Read the model definition and answer for the solid it produces. Units are mm, in the model's axes. A direction names the side the tool comes from. Give positions to 0.01 mm unless a question says otherwise; leave off trailing zeros. Loops run counter-clockwise (first coordinate to the right, second up) from the corner with the lowest first, then second, coordinate; pieces in that order, holes last. Notation, with made-up numbers: (-36.75, -34) - (17.25, -34) arc R13 ccw to (17.25, -21) - close; hole circle Ø1 at (8, 31). An arc over 180 degrees is marked (long way). Put each result on its own line as item: value. Start each with the question number.
1. Consider L1, parallel to X at y = -2.5, z = 5.1; L2, parallel to X at y = -17, z = 2.75; L3, parallel to X at y = -13, z = 0.95. Determine where each line is inside the solid, lowest interval first. Write a range as from..to.
2. For a pull along Y with two mould halves and no side action, classify faces 1 (the cylindrical face through (-15.43, 15.63, 0.74)), 2 (the flat face through (-12, 12, 0)) as released by +Y, released by -Y, zero draft, split by the parting line, or undercut.
3. For faces 3 (the cylindrical face through (14.151, -11.046, 3.782)), 4 (the cylindrical face through (-1.852, -21.386, 3.042)), determine the directions among +Z, -Z, +X, -X, +Y, -Y from which every point of the face is accessible in a straight line to the end or side of a thin tool.
4. Given pin 1 Ø12 at (x, y) = (-14, 8) entering from -Z; pin 2 Ø3.5 at (x, y) = (13.28, -14.95) entering from +Z; pin 3 Ø3 at (y, z) = (16.5, 4.5) entering from -X; pin 4 Ø1.5 at (y, z) = (5, 3) entering from +X, each flat-ended and moving along its own axis, determine where each tip first touches the part or whether it passes through.
5. A cutting plane is placed at B-B, the plane z = 4.3. Count the separate pieces of the cut face and the enclosed holes in it, plus the area to 3 significant figures.
6. A cutting plane is placed at A-A, the plane x = -14. Determine the outline of the cut face in (y, z), plus the area to 3 significant figures.
```python
from build123d import *

# Parameters (mm, degrees)
ESQUISSE5_R                                     = 27
ESQUISSE5_R_2                                   = 15
BASE_EXTRUSION_DEPTH                            = 6
TROU_TARAUD_M4X0_71_D                           = 3.3
R_P_TITION_CIRCULAIRE1_COUNT                    = 4
CHAMBRAGE_POUR_VIS_T_TE_CYLINDRIQUE_D           = 4.5
CHAMBRAGE_POUR_VIS_T_TE_CYLINDRIQUE_CBORE_D     = 8
CHAMBRAGE_POUR_VIS_T_TE_CYLINDRIQUE_CBORE_DEPTH = 4.5
R_P_TITION_CIRCULAIRE2_COUNT                    = 6


with BuildPart() as part:
    # Esquisse5 → Base-Extrusion (new body)
    with BuildSketch(Plane.XY):
        with Locations(Location((0, 0, 0), (0, 0, 180))):
            Circle(ESQUISSE5_R)
        with Locations(Location((0, 0, 0), (0, 0, 180))):
            Circle(ESQUISSE5_R_2, mode=Mode.SUBTRACT)
    extrude(amount=BASE_EXTRUSION_DEPTH)

    # Trou taraudé M4x0.71 (through all)
    with Locations(Plane(origin=(0, 0, 0), x_dir=(-1, 0, 0), z_dir=(0, 0, -1))):
        with Locations((22.959989216, 1.356058707)):
            trou_taraud_m4x0_71 = Hole(TROU_TARAUD_M4X0_71_D / 2)

    # Répétition circulaire1: Trou taraudé M4x0.71 ×4 about axis
    r_p_tition_circulaire1_axis = Axis((0, 0, 0), (0, 0, -1))
    for i in range(1, R_P_TITION_CIRCULAIRE1_COUNT):
        add(trou_taraud_m4x0_71.rotate(r_p_tition_circulaire1_axis, i * 360 / R_P_TITION_CIRCULAIRE1_COUNT), mode=Mode.SUBTRACT)

    # Chambrage pour vis à tête cylindrique à 6 pans creux (vis CHC) M41 (through all)
    with Locations(Plane.XY.offset(6)):
        with Locations((-13.28372675, 14.951341198)):
            chambrage_pour_vis_t_te_cylindrique = CounterBoreHole(CHAMBRAGE_POUR_VIS_T_TE_CYLINDRIQUE_D / 2, CHAMBRAGE_POUR_VIS_T_TE_CYLINDRIQUE_CBORE_D / 2, CHAMBRAGE_POUR_VIS_T_TE_CYLINDRIQUE_CBORE_DEPTH)

    # Répétition circulaire2: Chambrage pour vis à tête cylindrique à 6 pans creux (vis CHC) M41 ×6 about axis
    r_p_tition_circulaire2_axis = Axis((0, 0, 0), (0, 0, -1))
    for i in range(1, R_P_TITION_CIRCULAIRE2_COUNT):
        add(chambrage_pour_vis_t_te_cylindrique.rotate(r_p_tition_circulaire2_axis, i * 360 / R_P_TITION_CIRCULAIRE2_COUNT), mode=Mode.SUBTRACT)


solid = part.part
```
Return value:
1. L1: x = -26.88..-23.29, -15.89..-14.79, 14.79..21.77, 24.15..26.88
1. L2: x = -20.98..-9.78, -2.83..9.85, 16.72..20.98
1. L3: x = -23.66..-7.48, 7.48..12.16, 14.4..23.66
2. face 1: undercut
2. face 2: zero draft
3. face 3: +Z
3. face 4: +Z, -Z
4. pin 1: stops at z = 0
4. pin 2: passes through
4. pin 3: stops at x = -22.45
4. pin 4: stops at x = 26.66
5. separate pieces: 1
5. enclosed holes: 11
5. area: 1,250 mm2
6. outline: (-23.09, 0) - (-5.39, 0) - (-5.39, 6) - (-23.09, 6) - close; (5.39, 0) - (12.82, 0) - (12.82, 1.5) - (11.02, 1.5) - (11.02, 6) - (5.39, 6) - close; (17.08, 0) - (23.09, 0) - (23.09, 6) - (18.89, 6) - (18.89, 1.5) - (17.08, 1.5) - close
6. area: 171 mm2
